The listing builds one solid part. Answer for the finished solid, in the listing's coordinates (mm). Face numbers are marked on the shaded views. Coordinates: 2 decimals unless noted, no trailing zeros. Order: outer loops, then holes, each group sorted by start corner. A loop starts at its lowest first (then second) coordinate and runs counter-clockwise, first axis right, second up.
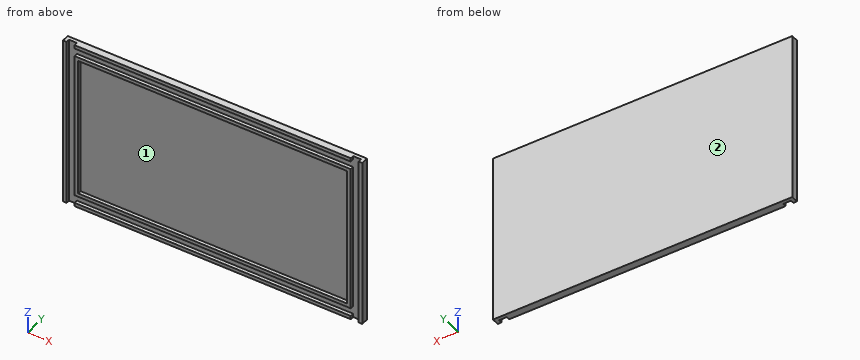
```python
from build123d import *

# Parameters (mm, degrees)
F0_W      = 2133.6
F0_H      = 1219.2
F1_DEPTH  = 25.4
F2_W      = 1968.5
F2_H      = 25.4
F3_DEPTH  = 25.4
F4_W      = 1968.5
F4_H      = 25.4
F5_DEPTH  = 25.4
F6_W      = 25.4
F6_H      = 1219.2
F7_DEPTH  = 25.4
F8_W      = 25.4
F8_H      = 1219.2
F9_DEPTH  = 25.4
F10_W     = 1968.5
F10_H     = 25.4
F11_DEPTH = 25.4
F12_W     = 1968.5
F12_H     = 25.4
F13_DEPTH = 25.4
F14_W     = 25.4
F14_H     = 1003.3
F15_DEPTH = 25.4
F16_W     = 25.4
F16_H     = 1003.3
F17_DEPTH = 25.4


with BuildPart() as f1:
    # F0 (on Front) → F1 (new body)
    with BuildSketch(Plane.XZ):
        with Locations((1066.8, 609.6)):
            Rectangle(F0_W, F0_H)
    extrude(amount=F1_DEPTH)

    # F2 (on face) → F3 (join)
    with BuildSketch(Plane.XZ.offset(25.4)):
        with Locations((1066.8, 1206.5)):
            Rectangle(F2_W, F2_H)
    extrude(amount=F3_DEPTH)

    # F4 (on face) → F5 (join)
    with BuildSketch(Plane.XZ.offset(25.4)):
        with Locations((1066.8, 12.7)):
            Rectangle(F4_W, F4_H)
    extrude(amount=F5_DEPTH)

    # F6 (on face) → F7 (join)
    with BuildSketch(Plane.XZ.offset(25.4)):
        with Locations((12.7, 609.6)):
            Rectangle(F6_W, F6_H)
    extrude(amount=F7_DEPTH)

    # F8 (on face) → F9 (join)
    with BuildSketch(Plane.XZ.offset(25.4)):
        with Locations((2120.9, 609.6)):
            Rectangle(F8_W, F8_H)
    extrude(amount=F9_DEPTH)

    # F10 (on face) → F11 (join)
    with BuildSketch(Plane.XZ.offset(25.4)):
        with Locations((1066.8, 1123.95)):
            Rectangle(F10_W, F10_H)
    extrude(amount=F11_DEPTH)

    # F12 (on face) → F13 (join)
    with BuildSketch(Plane.XZ.offset(25.4)):
        with Locations((1066.8, 95.25)):
            Rectangle(F12_W, F12_H)
    extrude(amount=F13_DEPTH)

    # F14 (on face) → F15 (join)
    with BuildSketch(Plane.XZ.offset(25.4)):
        with Locations((2038.35, 609.6)):
            Rectangle(F14_W, F14_H)
    extrude(amount=F15_DEPTH)

    # F16 (on face) → F17 (join)
    with BuildSketch(Plane.XZ.offset(25.4)):
        with Locations((95.25, 609.6)):
            Rectangle(F16_W, F16_H)
    extrude(amount=F17_DEPTH)


solid = f1.part
```
(1) Find section C-C (x = 767.5). Write down the section's boundary in (y, z), and give its area (3 significant figures).
(2) Find section B-B (z = 951.5). Write down the section's boundary in (x, y).
(3) Consider line 1 (Z direction, x = 1900, y = -26.5); line 2 (X direction, y = -29, z = 613); line 3 (Y direction, x = 352.5, z = 957). Determine where each line is inside the solid, lowest interval first.
(4) The mould has two halves that part along Z. Classify the marked faces 1 and 2: released by +Z, released by -Z, zero draft, split by the parting line, or undercut.
(5) Find section A-A (y = -33.5). Write down the section's boundary in (x, z), and give its area (3 significant figures).
Findings below:
1. outline: (-50.8, 0) - (0, 0) - (0, 1219.2) - (-50.8, 1219.2) - (-50.8, 1193.8) - (-25.4, 1193.8) - (-25.4, 1136.65) - (-50.8, 1136.65) - (-50.8, 1111.25) - (-25.4, 1111.25) - (-25.4, 107.95) - (-50.8, 107.95) - (-50.8, 82.55) - (-25.4, 82.55) - (-25.4, 25.4) - (-50.8, 25.4) - close
1. area: 33,500 mm2
2. outline: (0, -50.8) - (25.4, -50.8) - (25.4, -25.4) - (82.55, -25.4) - (82.55, -50.8) - (107.95, -50.8) - (107.95, -25.4) - (2025.65, -25.4) - (2025.65, -50.8) - (2051.05, -50.8) - (2051.05, -25.4) - (2108.2, -25.4) - (2108.2, -50.8) - (2133.6, -50.8) - (2133.6, 0) - (0, 0) - close
3. line 1: z = 0 to 25.4, 82.55 to 107.95, 1111.25 to 1136.65, 1193.8 to 1219.2
3. line 2: x = 0 to 25.4, 82.55 to 107.95, 2025.65 to 2051.05, 2108.2 to 2133.6
3. line 3: y = -25.4 to 0
4. face 1: undercut
4. face 2: zero draft
5. outline: (0, 0) - (25.4, 0) - (25.4, 1219.2) - (0, 1219.2) - close; (82.55, 0) - (2051.05, 0) - (2051.05, 25.4) - (82.55, 25.4) - close; (82.55, 82.55) - (2051.05, 82.55) - (2051.05, 1136.65) - (82.55, 1136.65) - close; (82.55, 1193.8) - (2051.05, 1193.8) - (2051.05, 1219.2) - (82.55, 1219.2) - close; (2108.2, 0) - (2133.6, 0) - (2133.6, 1219.2) - (2108.2, 1219.2) - close; hole (107.95, 107.95) - (2025.65, 107.95) - (2025.65, 1111.25) - (107.95, 1111.25) - close
5. area: 313,000 mm2
